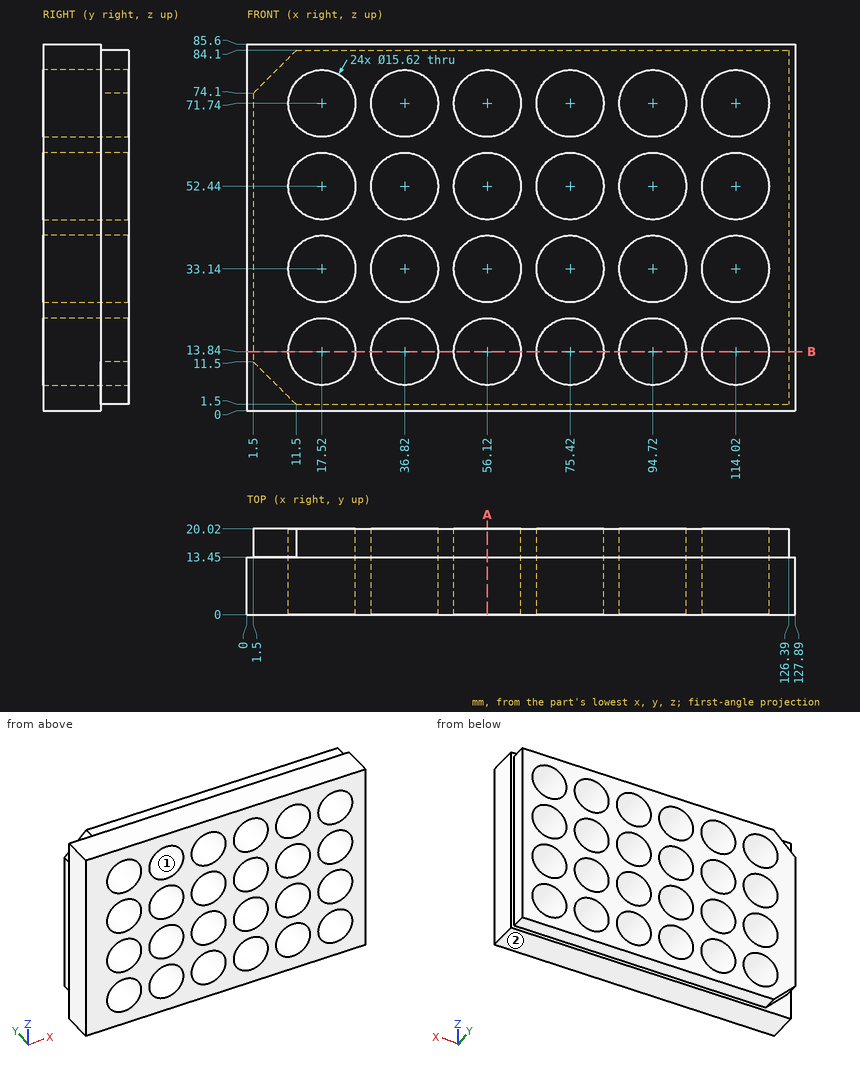
Source: three-view drawing plus pictorial views. Frame: mm from the lowest corner of the part. Round coordinates to 2 decimals unless told otherwise and drop trailing zeros. Loops run counter-clockwise (first coordinate to the right, second up) from the corner with the lowest first, then second, coordinate; pieces in that order, holes last.
1. Section query A-A on x = 56.12. Output: boundary loops of the cut face in (y, z).
2. Mould query, pull axis X, two halves, no side actions, for the marked faces 1 and 2. Classes: released by +X, released by -X, zero draft, split by the parting line, or undercut.
3. Ray query, L1, parallel to Z at x = 34, y = 12.5; L2, parallel to Z at x = 119, y = 18.5; L3, parallel to Y at x = 6.5, z = 5.5. Return the intervals inside material, ascending.
4. Contact query for a flat-ended pin moving along its axis: pin 1 (3.5 mm diameter, centred on y = 15.5, z = 57.5, fed in from -X). Output: stop coordinate, or through.
5. Section query B-B on z = 13.84. Give the number of separate pieces and of enclosed holes in the cut face, and give its area (3 significant figures).
Answers below:
1. outline: (0, 0) - (13.45, 0) - (13.45, 1.5) - (20.02, 1.5) - (20.02, 6.03) - (0, 6.03) - close; (0, 21.65) - (20.02, 21.65) - (20.02, 25.33) - (0, 25.33) - close; (0, 40.95) - (20.02, 40.95) - (20.02, 44.63) - (0, 44.63) - close; (0, 60.25) - (20.02, 60.25) - (20.02, 63.93) - (0, 63.93) - close; (0, 79.55) - (20.02, 79.55) - (20.02, 84.1) - (13.45, 84.1) - (13.45, 85.6) - (0, 85.6) - close
2. face 1: undercut
2. face 2: zero draft
3. L1: z = 0 to 6.56, 21.12 to 25.86, 40.42 to 45.16, 59.72 to 64.46, 79.02 to 85.6
3. L2: z = 1.5 to 7.82, 19.86 to 27.12, 39.16 to 46.42, 58.46 to 65.72, 77.76 to 84.1
3. L3: y = 0 to 13.45
4. pin 1: stops at x = 1.5
5. separate pieces: 7
5. enclosed holes: 0
5. area: 664 mm2
